```python
from build123d import *

# Parameters (mm, degrees)
SKETCH_2_W          = 1000
SKETCH_2_H          = 1160
EXTRUDE_1_DEPTH     = 16
CUT_EXTRUDE_1_DEPTH = 766.934723067


with BuildPart() as part:
    # 草图2 → 凸台-拉伸1 (new body)
    with BuildSketch(Plane.XY):
        Rectangle(SKETCH_2_W, SKETCH_2_H)
    extrude(amount=EXTRUDE_1_DEPTH)

    # 草图4 → 切除-拉伸1 (cut, through all)
    with BuildSketch(Plane(origin=(0, 0, 0), x_dir=(-1, 0, 0), z_dir=(0, 0, -1))):
        Polygon((-500, 360), (-430, 180), (-430, -180), (-500, -360), align=None)
        Polygon((430, 180), (430, -180), (500, -360), (500, 360), align=None)
    extrude(amount=-CUT_EXTRUDE_1_DEPTH, mode=Mode.SUBTRACT)


solid = part.part
```
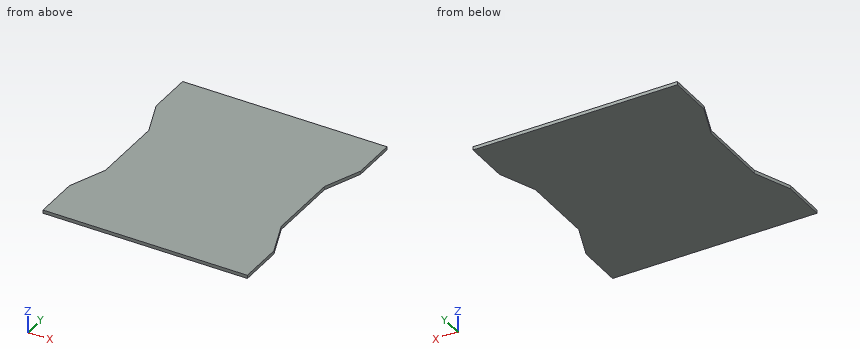
Check sheet for the modelled part. Datum: model origin and axes. Units: mm. Round coordinates to 2 decimals unless told otherwise and drop trailing zeros. Loops run counter-clockwise (first coordinate to the right, second up) from the corner with the lowest first, then second, coordinate; pieces in that order, holes last. Notation, with made-up numbers: (5.5, 23) - (52.5, 23) arc R18 cw to (52.5, 30) - close; hole circle Ø7 at (46, 55). An arc over 180 degrees is marked (long way). Write item = value, one per line. Start each with the question number.
Q1. Section check B-B (y = 96.5). Record the boundary of the cut face in (x, z).
Q2. Thickness scan on L1, parallel to X at y = -25, z = 13.5; L2, parallel to X at y = 254, z = 1.75. Record the ranges inside material, lowest first.
Q3. Section check C-C (y = -198.5). Record the boundary of the cut face in (x, z), plus the area to 3 significant figures.
Q4. Depth check by flat-ended pin: P1, Ø4, axis at y = -188.5, z = 4, coming from the -X side; P2, Ø8, axis at y = 42, z = 8, coming from the +X side; P3, Ø4, axis at y = 12.5, z = 5.5, coming from the -X side. Enter the tip coordinate at first touch or a pass-through.
Q5. Section check A-A (z = 2.5). Record the boundary of the cut face in (x, y).
Derived:
q1.outline = (-430, 0) - (430, 0) - (430, 16) - (-430, 16) - close
q2.L1 = -430 to 430
q2.L2 = -458.78 to 458.78
q3.outline = (-437.19, 0) - (437.19, 0) - (437.19, 16) - (-437.19, 16) - close
q3.area = 14,000 mm^2
q4.P1 = -434.08
q4.P2 = 430
q4.P3 = -430
q5.outline = (-500, -580) - (500, -580) - (500, -360) - (430, -180) - (430, 180) - (500, 360) - (500, 580) - (-500, 580) - (-500, 360) - (-430, 180) - (-430, -180) - (-500, -360) - close
